from build123d import *

# Parameters (mm, degrees)
SKETCH1_W                 = 48
SKETCH1_H                 = 12
BOSS_EXTRUDE2_DEPTH       = 4
SKETCH3_R                 = 3.25
BOSS_EXTRUDE3_DEPTH       = 2
SKETCH4_R                 = 3.85
BOSS_EXTRUDE4_DEPTH       = 3.3
SKETCH5_W                 = 10.744623103
SKETCH5_H                 = 3.104002229
SKETCH5_W_2               = 12.040799858
SKETCH5_H_2               = 4.707168217
CUT_EXTRUDE6_DEPTH        = 1.6
SKETCH6_R                 = 2.1
CUT_EXTRUDE7_DEPTH        = 1.6
BOSS_EXTRUDE5_DEPTH       = 48
SKETCH11_R                = 2
CUT_EXTRUDE12_DEPTH       = 46.960925441
CUT_EXTRUDE13_START       = -3.247821806
CUT_EXTRUDE13_OUTLINE_R   = 3.036171251
CUT_EXTRUDE13_OUTLINE_R_2 = 2
CUT_EXTRUDE13_OUTLINE_R_3 = 3.150431912
CUT_EXTRUDE13_DEPTH       = 6.452188627


# Read off the part's stored shape, not the designer's step: Cut-Extrude13
with BuildPart() as part:
    # Sketch1 → Boss-Extrude2 (new body)
    with BuildSketch(Plane(origin=(0, 0, 0), x_dir=(1, 0, 0), z_dir=(0, 1, 0))):
        with Locations((-18.755819717, 5.963784416)):
            Rectangle(SKETCH1_W, SKETCH1_H)
    extrude(amount=BOSS_EXTRUDE2_DEPTH)

    # Sketch3 → Boss-Extrude3 (add)
    with BuildSketch(Plane(origin=(0, 4, 0), x_dir=(1, 0, 0), z_dir=(0, 1, 0))):
        with Locations(Location((-18.755819717, 5.963784416, 0), (0, 0, 270))):
            Circle(SKETCH3_R)
    extrude(amount=BOSS_EXTRUDE3_DEPTH)

    # Sketch4 → Boss-Extrude4 (add)
    with BuildSketch(Plane(origin=(0, 6, 0), x_dir=(1, 0, 0), z_dir=(0, 1, 0))):
        with Locations(Location((-18.755819717, 5.963784416, 0), (0, 0, 270))):
            Circle(SKETCH4_R)
    extrude(amount=BOSS_EXTRUDE4_DEPTH)

    # Sketch5 → Cut-Extrude6 (cut)
    with BuildSketch(Plane(origin=(0, 9.3, 0), x_dir=(1, 0, 0), z_dir=(0, 1, 0))):
        with Locations((-18.784487645, 3.131783302)):
            Rectangle(SKETCH5_W, SKETCH5_H)
        with Locations((-18.682157901, 9.597368525)):
            Rectangle(SKETCH5_W_2, SKETCH5_H_2)
    extrude(amount=-CUT_EXTRUDE6_DEPTH, mode=Mode.SUBTRACT)

    # Sketch6 → Cut-Extrude7 (cut)
    with BuildSketch(Plane(origin=(0, 9.3, 0), x_dir=(1, 0, 0), z_dir=(0, 1, 0))):
        with Locations((-18.755819717, 5.963784416)):
            Circle(SKETCH6_R)
    extrude(amount=-CUT_EXTRUDE7_DEPTH, mode=Mode.SUBTRACT)

    # Sketch7 → Boss-Extrude5 (add)
    with BuildSketch(Plane(origin=(5.244180283, 0, 0), x_dir=(0, 0, -1), z_dir=(1, 0, 0))):
        Polygon((11.963784416, 0), (0, -9.109804798), (-0.036215584, 0), align=None)
    extrude(amount=-BOSS_EXTRUDE5_DEPTH)

    # Sketch11 → Cut-Extrude12 (cut, through all)
    with BuildSketch(Plane(origin=(0, -5.766415649, -4.390828112), x_dir=(1, 0, 0), z_dir=(0, -0.7956067081089262, -0.6058134746042532))):
        with Locations(Location((0.874180283, -1.977052592, 0), (0, 0, 270))):
            Circle(SKETCH11_R)
        with Locations(Location((-38.525819717, -1.977052592, 0), (0, 0, 270))):
            Circle(SKETCH11_R)
    extrude(amount=-CUT_EXTRUDE12_DEPTH, mode=Mode.SUBTRACT)

    # Cut-Extrude13 outline → Cut-Extrude13 (cut)
    # profile 1 of 2: a face of its own
    with BuildSketch(Plane(origin=(0, 0, 0), x_dir=(1, 0, 0), z_dir=(0, 0.7956067081089261, 0.6058134746042532)).offset(CUT_EXTRUDE13_START)):
        with Locations((-38.643729383, 2.019534021)):
            Circle(CUT_EXTRUDE13_OUTLINE_R)
        with Locations((-38.525819717, 1.977052592)):
            Circle(CUT_EXTRUDE13_OUTLINE_R_2, mode=Mode.SUBTRACT)
    # profile 2 of 2: a face of its own
    with BuildSketch(Plane(origin=(0, 0, 0), x_dir=(1, 0, 0), z_dir=(0, 0.7956067081089261, 0.6058134746042532)).offset(CUT_EXTRUDE13_START)):
        with Locations((0.730306236, 2.019534021)):
            Circle(CUT_EXTRUDE13_OUTLINE_R_3)
        with Locations((0.874180283, 1.977052592)):
            Circle(CUT_EXTRUDE13_OUTLINE_R_2, mode=Mode.SUBTRACT)
    extrude(amount=CUT_EXTRUDE13_DEPTH, mode=Mode.SUBTRACT)


solid = part.part
The listing builds one solid part. Answer for the finished solid, in the listing's coordinates (mm). A direction names the side the tool comes from. Round coordinates to 2 decimals unless told otherwise and drop trailing zeros. Write each loop counter-clockwise with the first axis right and the second up, starting at its lowest first coordinate (ties: lowest second). Pieces come first, ordered by that corner, then holes. Notation, with made-up numbers: M 56.5,40 L 60.5,40 A16 ccw 60.5,49 Z; hole C 34,-19.5 d6. An arc over 180 degrees is marked long. Write each question's results on one line, items separated by ' | '. Start each with the question number.
Item 1: Straight lines are drawn through the part: probe 1 along X at (y, z) = (-4, -4.5); probe 2 along X at (y, z) = (0.75, -2.5); probe 3 along Z at (x, y) = (-36, -0.75). For each, find the intervals that lie inside material, in ascending order.
Item 2: Given pin 1 Ø3 at (x, y) = (-6.5, -4) entering from +Z; pin 2 Ø6 at (x, z) = (-18.5, -6) entering from +Y; pin 3 Ø0.5 at (x, y) = (-21.5, 8) entering from -Z; pin 4 Ø2 at (x, y) = (-14.5, 6) entering from -Z, each flat-ended and moving along its own axis, determine where each tip first touches the part or whether it passes through.
Item 3: Find section C-C on y = 7. Write down the section's boundary in (x, z), and give its area (3 significant figures).
Item 4: Which of the six approach directions +Z, -Z, +X, -X, +Y, -Y give full straight-line access (tool end or side, diameter ignored) to faces 5 (the flat face through (-42.756, -1, -5)), 6 (the cylindrical face through (-20.856, 8.511, -5.983)), 7 (the flat face through (-16, 9, -4.684)), 8 (the flat face through (-19, 2, 0.036)), 9 (the flat face through (-21, 9, -7.244))?
Item 5: Find section A-A on x = -3.5. Write down the section's boundary in (y, z), and give its area (3 significant figures).
Item 6: Find section B-B on z = -8. Write down the section's boundary in (x, y).
Item 7: Find section D-D on z = -10.75. Write down the section's boundary in (x, y).
Item 8: The mould has two halves that part along X. Classify faces 1 (the cylindrical face through (-21.93, 4.99, -6.67)), 2 (the flat face through (-16, 9.3, -6)), 3 (the cylindrical face through (-36.543, -3.157, -4.562)), 4 (the flat face through (-0.014, -2.606, -1.938)): +X half, -X half, draft (parallel to the pull), parting line (faces both ways), or undercut.
Answer block:
1) probe 1: x = -42.76 to -40.35, -36.7 to -0.95, 2.7 to 5.24 | probe 2: x = -42.76 to -41.65, -35.64 to -2.39, 3.85 to 5.24 | probe 3: z = -10.98 to -4.38, -1.23 to 0.03
2) pin 1: stops at z = 0.03 | pin 2: stops at y = 9.3 | pin 3: stops at z = -7.24 | pin 4: stops at z = -8.02
3) outline: C -18.76,-5.96 d7.7 | area: 46.6 mm²
4) face 5: +Z, -Z, -X, +Y, -Y | face 6: +Y | face 7: +Z, +X, -X, +Y | face 8: +Z, +X, -X, +Y, -Y | face 9: -Z, +X, -X, +Y
5) outline: M -9.11,0 L 0,-11.96 L 4,-11.96 L 4,0.04 L 0,0.04 Z | area: 103 mm²
6) outline: M -42.76,-3.02 L 5.24,-3.02 L 5.24,4 L -16.22,4 L -16.22,6 L -15.49,6 L -15.49,7.7 L -22.02,7.7 L -22.02,6 L -21.29,6 L -21.29,4 L -42.76,4 Z
7) outline: M -42.76,-0.92 L 5.24,-0.92 L 5.24,4 L -42.76,4 Z
8) face 1: parting line | face 2: draft | face 3: undercut | face 4: undercut
